For this review, take the finished solid that the model builds, in its own axes (mm). A direction names the side the tool comes from. Coordinates: 2 decimals unless noted, no trailing zeros. Write each loop counter-clockwise with the first axis right and the second up, starting at its lowest first coordinate (ties: lowest second). Pieces come first, ordered by that corner, then holes.
```python
from build123d import *

# Parameters (mm, degrees)
EXTRUDE_1_DEPTH     = 3
SKETCH_2_R          = 1.5
CUT_EXTRUDE_1_DEPTH = 3
CHAMFER_1_SIZE      = 0.5
FILLET_1_R          = 2


with BuildPart() as part:
    # 草图1 → 凸台-拉伸1 (new body)
    with BuildSketch(Plane(origin=(0, 0, 0), x_dir=(0, 0, -1), z_dir=(1, 0, 0))):
        Polygon((25, 25), (-25, 25), (-25, 17.5), (-7.5, 17.5), (-7.5, -17.5), (-25, -17.5), (-25, -25), (25, -25), (25, -17.5), (7.5, -17.5), (7.5, 17.5), (25, 17.5), align=None)
    extrude(amount=EXTRUDE_1_DEPTH)

    # 草图2 → 切除-拉伸1 (cut)
    with BuildSketch(Plane(origin=(3, 0, 0), x_dir=(0, 0, -1), z_dir=(1, 0, 0))):
        with Locations((-21, 21)):
            Circle(SKETCH_2_R)
        with Locations((-21, -21)):
            Circle(SKETCH_2_R)
        with Locations(Location((21, -21, 0), (0, 0, 180))):
            Circle(SKETCH_2_R)
        with Locations(Location((21, 21, 0), (0, 0, 180))):
            Circle(SKETCH_2_R)
    extrude(amount=-CUT_EXTRUDE_1_DEPTH, mode=Mode.SUBTRACT)

    # 倒角1
    chamfer_1_edges = [part.edges().sort_by_distance(p)[0] for p in [
        (3, 21, -22.5),
        (3, -21, -22.5),
        (3, -21, 22.5),
        (3, 21, 22.5),
    ]]
    chamfer(chamfer_1_edges, length=CHAMFER_1_SIZE)

    # 圆角1
    fillet_1_edges = [part.edges().sort_by_distance(p)[0] for p in [
        (1.5, 25, 25),
        (1.5, 25, -25),
        (1.5, 17.5, -25),
        (1.5, -17.5, -25),
        (1.5, -25, -25),
        (1.5, -25, 25),
        (1.5, -17.5, 25),
        (1.5, 17.5, 25),
    ]]
    fillet(fillet_1_edges, radius=FILLET_1_R)


solid = part.part
```
1) For L1, parallel to Y at x = 1.35, z = 21; L2, parallel to Y at x = 0.5, z = -10; L3, parallel to Y at x = 2.25, z = 20.5, list the stretches that pass through material, from the lowest coordinate up.
2) Clearance check with flat-ended pins moving along their axes: P1, Ø0.9, axis at x = 1.5, y = -7.5, coming from the -Z side; P2, Ø1.5, axis at x = 1.5, y = 8.5, coming from the +Z side. State where each tip first meets the part, or that it passes through.
3) Consider section C-C (y = -21). Give the boundary of the cut face in (x, z).
4) Consider section B-B (x = 0.9). Give the boundary of the cut face in (y, z).
5) The part is to be moulded in two halves that separate along Z. For faces 1 (the face through (1, 21, -25)), 2 (the face through (1.27, 19.99, -22.11)), 3 (the face through (1, -21, 25)), say which applies: pulls with the +Z half, pulls with the -Z half, needs draft (parallel to the pull), parting line crosses it, or undercut.
6) Tool access review of faces 4 (the face through (1, 0, -7.5)), 5 (the face through (1.52, 18.1, 24.43)), 6 (the face through (0, 0, 0)): name each direction out of +Z, -Z, +X, -X, +Y, -Y from which nothing blocks a thin tool from reaching the whole face with its end or side.
7) Consider section D-D (z = -13). Give the boundary of the cut face in (x, y), then the cut area to 3 significant figures.
8) Consider section A-A (z = -21). Give the boundary of the cut face in (x, y), then the cut area to 3 significant figures.
Results:
1. L1: y = -25 to -22.5, -19.5 to -17.5, 17.5 to 19.5, 22.5 to 25
1. L2: y = -25 to -17.5, 17.5 to 25
1. L3: y = -25 to -22.41, -19.59 to -17.5, 17.5 to 19.59, 22.41 to 25
2. P1: stops at z = -7.5
2. P2: stops at z = 7.5
3. outline: (0, -25) - (3, -25) - (3, -23) - (2.5, -22.5) - (0, -22.5) - close; (0, -19.5) - (2.5, -19.5) - (3, -19) - (3, 19) - (2.5, 19.5) - (0, 19.5) - close; (0, 22.5) - (2.5, 22.5) - (3, 23) - (3, 25) - (0, 25) - close
4. outline: (-25, -23) arc R2 ccw to (-23, -25) - (-19.5, -25) arc R2 ccw to (-17.5, -23) - (-17.5, -7.5) - (17.5, -7.5) - (17.5, -23) arc R2 ccw to (19.5, -25) - (23, -25) arc R2 ccw to (25, -23) - (25, 23) arc R2 ccw to (23, 25) - (19.5, 25) arc R2 ccw to (17.5, 23) - (17.5, 7.5) - (-17.5, 7.5) - (-17.5, 23) arc R2 ccw to (-19.5, 25) - (-23, 25) arc R2 ccw to (-25, 23) - close; hole circle Ø3 at (-21, -21); hole circle Ø3 at (-21, 21); hole circle Ø3 at (21, -21); hole circle Ø3 at (21, 21)
5. face 1: pulls with the -Z half
5. face 2: undercut
5. face 3: pulls with the +Z half
6. face 4: -Z, +X, -X
6. face 5: +Z, +X, -X
6. face 6: +Z, -Z, -X, +Y, -Y
7. outline: (0, -25) - (3, -25) - (3, -17.5) - (0, -17.5) - close; (0, 17.5) - (3, 17.5) - (3, 25) - (0, 25) - close
7. area: 45.0 mm2
8. outline: (0, -25) - (3, -25) - (3, -23) - (2.5, -22.5) - (0, -22.5) - close; (0, -19.5) - (2.5, -19.5) - (3, -19) - (3, -17.5) - (0, -17.5) - close; (0, 17.5) - (3, 17.5) - (3, 19) - (2.5, 19.5) - (0, 19.5) - close; (0, 22.5) - (2.5, 22.5) - (3, 23) - (3, 25) - (0, 25) - close
8. area: 26.5 mm2
